from build123d import *

# Parameters (mm, degrees)
SKETCH1_R           = 30.315
SKETCH1_R_2         = 27.955876632
BOSS_EXTRUDE1_DEPTH = 2.54
BOSS_EXTRUDE3_DEPTH = 2.54


with BuildPart() as part:
    # Sketch1 → Boss-Extrude1 (new body)
    with BuildSketch(Plane(origin=(0, 0, 0), x_dir=(1, 0, 0), z_dir=(0, 1, 0))):
        Circle(SKETCH1_R)
        Circle(SKETCH1_R_2, mode=Mode.SUBTRACT)
    extrude(amount=BOSS_EXTRUDE1_DEPTH)

    # Sketch2 → Boss-Extrude3 (add)
    with BuildSketch(Plane(origin=(0, 2.54, 0), x_dir=(1, 0, 0), z_dir=(0, 1, 0))):
        with BuildLine():
            ThreePointArc((23.249475333, 15.523947146), (22.126610026, 17.086373723), (20.89893406, 18.567864536))
            Line((20.89893406, 18.567864536), (-18.197502423, -21.222204028))
            ThreePointArc((-18.197502423, -21.222204028), (-16.694652957, -22.423639332), (-15.112723253, -23.51885699))
            Line((-15.112723253, -23.51885699), (23.249475333, 15.523947146))
        make_face()
        with BuildLine():
            ThreePointArc((26.276234192, 9.544137201), (25.507547042, 11.440982568), (24.602142837, 13.276505792))
            Line((24.602142837, 13.276505792), (-12.841843795, -24.831795871))
            ThreePointArc((-12.841843795, -24.831795871), (-10.990683551, -25.70478386), (-9.080614707, -26.439997632))
            Line((-9.080614707, -26.439997632), (26.276234192, 9.544137201))
        make_face()
        with BuildLine():
            ThreePointArc((27.875984112, 2.112000943), (27.597491722, 4.462005025), (27.121248921, 6.780036517))
            Line((27.121248921, 6.780036517), (-6.302082474, -27.236277181))
            ThreePointArc((-6.302082474, -27.236277181), (-3.97603503, -27.671685595), (-1.621497222, -27.908811959))
            Line((-1.621497222, -27.908811959), (27.875984112, 2.112000943))
        make_face()
        with BuildLine():
            ThreePointArc((26.762200244, -8.081811449), (27.538835575, -4.810776795), (27.917192699, -1.470166667))
            Line((27.917192699, -1.470166667), (1.960841153, -27.887024584))
            ThreePointArc((1.960841153, -27.887024584), (5.294281665, -27.449983968), (8.551154051, -26.615950154))
            Line((8.551154051, -26.615950154), (26.762200244, -8.081811449))
        make_face()
        with BuildLine():
            ThreePointArc((15.229009426, -23.443726455), (19.940833039, -19.593218621), (23.707891831, -14.814415383))
            Line((23.707891831, -14.814415383), (15.229009426, -23.443726455))
        make_face()
        with BuildLine():
            ThreePointArc((16.305164724, 22.708426665), (15.714169419, 23.121330362), (15.112723252, 23.518856991))
            Line((15.112723252, 23.518856991), (-23.249475334, -15.523947145))
            ThreePointArc((-23.249475334, -15.523947145), (-22.982270651, -15.916855029), (-22.708426665, -16.305164724))
            ThreePointArc((-22.708426665, -16.305164724), (-22.41820217, -16.701953471), (-22.121045331, -17.0935775))
            ThreePointArc((-22.121045331, -17.0935775), (-21.522616878, -17.841188329), (-20.898934061, -18.567864535))
            Line((-20.898934061, -18.567864535), (18.197502422, 21.222204029))
            ThreePointArc((18.197502422, 21.222204029), (17.651262262, 21.678652606), (17.0935775, 22.121045331))
            ThreePointArc((17.0935775, 22.121045331), (16.701953471, 22.41820217), (16.305164724, 22.708426665))
        make_face()
        with BuildLine():
            ThreePointArc((12.841843795, 24.831795872), (10.99068355, 25.704783861), (9.080614706, 26.439997633))
            Line((9.080614706, 26.439997633), (-26.276234193, -9.544137201))
            ThreePointArc((-26.276234193, -9.544137201), (-25.507547043, -11.440982567), (-24.602142838, -13.276505791))
            Line((-24.602142838, -13.276505791), (12.841843795, 24.831795872))
        make_face()
        with BuildLine():
            ThreePointArc((3.386258142, 27.750032325), (2.505135962, 27.843407336), (1.621497221, 27.90881196))
            Line((1.621497221, 27.90881196), (-27.875984113, -2.112000942))
            ThreePointArc((-27.875984113, -2.112000942), (-27.820304798, -2.74985076), (-27.750032325, -3.386258142))
            ThreePointArc((-27.750032325, -3.386258142), (-27.488066672, -5.092860582), (-27.121248922, -6.780036516))
            Line((-27.121248922, -6.780036516), (6.302082473, 27.236277182))
            ThreePointArc((6.302082473, 27.236277182), (4.850976402, 27.531782837), (3.386258142, 27.750032325))
        make_face()
        with BuildLine():
            Line((-27.9171927, 1.470166667), (-1.960841154, 27.887024585))
            ThreePointArc((-1.960841154, 27.887024585), (-5.294281666, 27.449983969), (-8.551154052, 26.615950155))
            Line((-8.551154052, 26.615950155), (-26.762200245, 8.08181145))
            ThreePointArc((-26.762200245, 8.08181145), (-27.538835576, 4.810776796), (-27.9171927, 1.470166667))
        make_face()
        with BuildLine():
            Line((-23.707891832, 14.814415383), (-15.229009427, 23.443726455))
            ThreePointArc((-15.229009427, 23.443726455), (-19.940833039, 19.593218621), (-23.707891832, 14.814415383))
        make_face()
    extrude(amount=-BOSS_EXTRUDE3_DEPTH)


solid = part.part
Build history of the part. All positions in model axes, mm. Coordinates: 2 decimals unless noted, no trailing zeros. Write each loop counter-clockwise with the first axis right and the second up, starting at its lowest first coordinate (ties: lowest second). Pieces come first, ordered by that corner, then holes.
(1) Drill centre lines: line 1 (X direction, y = 0.4, z = -18.5); line 2 (X direction, y = 0.65, z = -22); line 3 (X direction, y = 0.3, z = -19). Where is each one in solid material? Low to high.
(2) Mould opens along Z. For faces 1 (the cylindrical face through (28.003, 1.252, 11.611)), 2 (the cylindrical face through (0.145, 1.252, 27.956)), 3 (the flat face through (0, 2.54, 6)) say: pulls with the +Z half, pulls with the -Z half, needs draft (parallel to the pull), parting line crosses it, or undercut.
(3) Cut at C-C on z = 0. State how many separate pieces and enclosed holes the cut face has, and give its area (3 significant figures).
(4) Cut at B-B on x = -3.5. List the corners of the cut face in (y, z), and give its area (3 significant figures).
(5) Pin check, flat tips, straight feed: pin 1 Ø1.5 at (y, z) = (2, 19) entering from -X; pin 2 Ø1.5 at (x, y) = (17.5, 1) entering from +Z. Stop position of each tip, or through.
(6) Cut at A-A on x = -19.5. List the corners of the cut face in (y, z).
Working result:
1. line 1: x = -24.02 to -20.09, -16.53 to -11.18, -7.62 to -2.28, 1.28 to 6.62, 10.18 to 15.52, 20.83 to 24.02
1. line 2: x = -20.86 to -16.65, -13.09 to -7.75, -4.18 to 1.16, 4.72 to 10.06, 13.62 to 20.86
1. line 3: x = -23.62 to -19.6, -16.03 to -10.69, -7.13 to -1.79, 1.77 to 7.11, 10.67 to 16.01, 20.51 to 23.62
2. face 1: parting line crosses it
2. face 2: undercut
2. face 3: needs draft
3. separate pieces: 8
3. enclosed holes: 0
3. area: 93.4 mm2
4. outline: (0, -30.11) - (2.54, -30.11) - (2.54, -26.32) - (0, -26.32) - close; (0, -22.7) - (2.54, -22.7) - (2.54, -17.26) - (0, -17.26) - close; (0, -13.64) - (2.54, -13.64) - (2.54, -8.2) - (0, -8.2) - close; (0, -4.58) - (2.54, -4.58) - (2.54, 0.86) - (0, 0.86) - close; (0, 6.26) - (2.54, 6.26) - (2.54, 11.7) - (0, 11.7) - close; (0, 15.32) - (2.54, 15.32) - (2.54, 20.76) - (0, 20.76) - close; (0, 24.38) - (2.54, 24.38) - (2.54, 30.11) - (0, 30.11) - close
4. area: 93.2 mm2
5. pin 1: stops at x = -24.21
5. pin 2: stops at z = 25.27
6. outline: (0, -23.21) - (2.54, -23.21) - (2.54, -19.1) - (0, -19.1) - close; (0, -15.47) - (2.54, -15.47) - (2.54, -10.04) - (0, -10.04) - close; (0, -6.41) - (2.54, -6.41) - (2.54, -0.98) - (0, -0.98) - close; (0, 2.65) - (2.54, 2.65) - (2.54, 8.08) - (0, 8.08) - close; (0, 11.71) - (2.54, 11.71) - (2.54, 17.14) - (0, 17.14) - close; (0, 20.03) - (2.54, 20.03) - (2.54, 23.21) - (0, 23.21) - close
